Design review of the part built by this model. Coordinates are the model's own, in mm. A direction names the side the tool comes from. Give positions to 0.01 mm unless a question says otherwise; leave off trailing zeros. Loops run counter-clockwise (first coordinate to the right, second up) from the corner with the lowest first, then second, coordinate; pieces in that order, holes last. Notation, with made-up numbers: M 39.5,21.5 L 89.5,21.5 A20 cw 89.5,25.5 Z; hole C -28,-30.75 d1. An arc over 180 degrees is marked long. Answer as CSV lines item,"result".
```python
from build123d import *

# Parameters (mm, degrees)
BOSS_EXTRUDE1_DEPTH = 75
BOSS_EXTRUDE2_START = 225
BOSS_EXTRUDE2_DEPTH = 75
BOSS_EXTRUDE4_START = 75
BOSS_EXTRUDE4_DEPTH = 75
BOSS_EXTRUDE5_DEPTH = 75


# Read off the part's stored shape, not the designer's step: Boss-Extrude4
with BuildPart() as part:
    # Sketch2 → Boss-Extrude1 (new body)
    with BuildSketch(Plane(origin=(0, 0, 0), x_dir=(1, 0, 0), z_dir=(0, 1, 0))):
        with BuildLine():
            ThreePointArc((45, 244.20687951), (47.800691376, 236.146227949), (54.996015936, 231.558714436))
            ThreePointArc((54.996015936, 231.558714436), (116.038816401, 207.795555988), (168.291413922, 168.291413922))
            Line((168.291413922, 168.291413922), (141.421356237, 141.421356237))
            ThreePointArc((141.421356237, 141.421356237), (0, 200), (-141.421356237, 141.421356237))
            Line((-141.421356237, 141.421356237), (-168.291413922, 168.291413922))
            ThreePointArc((-168.291413922, 168.291413922), (-116.038816401, 207.795555988), (-54.996015936, 231.558714436))
            ThreePointArc((-54.996015936, 231.558714436), (-47.800691376, 236.146227949), (-45, 244.20687951))
            Line((-45, 244.20687951), (-45, 275))
            Line((-45, 275), (45, 275))
            Line((45, 275), (45, 244.20687951))
        make_face()
    extrude(amount=BOSS_EXTRUDE1_DEPTH)



with BuildPart() as body_2:
    # Sketch2_3 → Boss-Extrude2 (new body)
    with BuildSketch(Plane(origin=(0, 0, 0), x_dir=(1, 0, 0), z_dir=(0, 1, 0)).offset(BOSS_EXTRUDE2_START)):
        with BuildLine():
            Line((141.421356237, 141.421356237), (168.291413922, 168.291413922))
            ThreePointArc((168.291413922, 168.291413922), (116.038816401, 207.795555988), (54.996015936, 231.558714436))
            ThreePointArc((54.996015936, 231.558714436), (47.800691376, 236.146227949), (45, 244.20687951))
            Line((45, 244.20687951), (45, 275))
            Line((45, 275), (-45, 275))
            Line((-45, 275), (-45, 244.20687951))
            ThreePointArc((-45, 244.20687951), (-47.800691376, 236.146227949), (-54.996015936, 231.558714436))
            ThreePointArc((-54.996015936, 231.558714436), (-116.038816401, 207.795555988), (-168.291413922, 168.291413922))
            Line((-168.291413922, 168.291413922), (-141.421356237, 141.421356237))
            ThreePointArc((-141.421356237, 141.421356237), (0, 200), (141.421356237, 141.421356237))
        make_face()
    extrude(amount=-BOSS_EXTRUDE2_DEPTH)


with BuildPart() as part_1:
    add(part.part)

    add(body_2.part)  # Boss-Extrude4 merges body 2
    # Boss-Extrude4 outline → Boss-Extrude4 (add)
    with BuildSketch(Plane(origin=(0, 0, 0), x_dir=(1, 0, 0), z_dir=(0, 1, 0)).offset(BOSS_EXTRUDE4_START)):
        with BuildLine():
            Line((45, 194.871752699), (45, 275))
            Line((45, 275), (-45, 275))
            Line((-45, 275), (-45, 194.871752699))
            ThreePointArc((-45, 194.871752699), (0, 200), (45, 194.871752699))
        make_face()
    extrude(amount=BOSS_EXTRUDE4_DEPTH)

    # Sketch4_6 → Boss-Extrude5 (add)
    with BuildSketch(Plane(origin=(0, 0, -275), x_dir=(-1, 0, 0), z_dir=(0, 0, -1))):
        with BuildLine():
            ThreePointArc((37.5, 169), (-9.845373608, 205.18450799), (-32.330326321, 150))
            Line((-32.330326321, 150), (32.330326321, 150))
            ThreePointArc((32.330326321, 150), (36.18450799, 159.154626392), (37.5, 169))
        make_face()
        with BuildLine():
            Line((32.330326321, 150), (-32.330326321, 150))
            ThreePointArc((-32.330326321, 150), (0, 131.5), (32.330326321, 150))
        make_face()
        with BuildLine():
            ThreePointArc((32.330326321, 75), (0, 93.5), (-32.330326321, 75))
            Line((-32.330326321, 75), (32.330326321, 75))
        make_face()
        with BuildLine():
            Line((32.330326321, 75), (-32.330326321, 75))
            ThreePointArc((-32.330326321, 75), (-9.845373608, 19.81549201), (37.5, 56))
            ThreePointArc((37.5, 56), (36.18450799, 65.845373608), (32.330326321, 75))
        make_face()
    extrude(amount=BOSS_EXTRUDE5_DEPTH)


solid = part_1.part
```
1. We need section A-A, the plane x = 62. Write out the cut boundary in (y, z), plus the area to 3 significant figures.
Answer block:
outline,"M 0,-229.78 L 75,-229.78 L 75,-190.15 L 0,-190.15 Z; M 150,-229.78 L 225,-229.78 L 225,-190.15 L 150,-190.15 Z"
area,"5,950 mm²"
2. To check wall thickness, follow L1, parallel to Y at x = -10.5, z = -304; L2, parallel to X at y = 28, z = -169.5; L3, parallel to X at y = 97.5, z = -264.5. State the ranges of each line that lie inside material, in increasing order. Write a range as [from, to].
Answer block:
L1,"[20, 92], [133, 205]"
L2,"[-167.07, -106.16], [106.16, 167.07]"
L3,"[-45, 45]"
3. The part is to be moulded in two halves that separate along Y. For faces 1 (the flat face through (-2, 225, -209)), 2 (the flat face through (108, 75, -194)), 3 (the flat face through (2, 0, -209)), 4 (the flat face through (-155, 37, -155)), say which applies: pulls with the +Y half, pulls with the -Y half, needs draft (parallel to the pull), parting line crosses it, or undercut.
Answer block:
face 1,"pulls with the +Y half"
face 2,"undercut"
face 3,"pulls with the -Y half"
face 4,"needs draft"
4. We need section C-C, the plane y = 70. Write out the cut boundary in (x, z).
Answer block:
outline,"M -168.29,-168.29 A238 ccw -55,-231.56 A13 cw -45,-244.21 L -45,-275 L -34.79,-275 L -34.79,-350 L 34.79,-350 L 34.79,-275 L 45,-275 L 45,-244.21 A13 cw 55,-231.56 A238 ccw 168.29,-168.29 L 141.42,-141.42 A200 cw -141.42,-141.42 Z"
5. We need section D-D, the plane x = 0. Write out the cut boundary in (y, z), plus the area to 3 significant figures.
Answer block:
outline,"M 0,-275 L 18.5,-275 L 18.5,-350 L 93.5,-350 L 93.5,-275 L 131.5,-275 L 131.5,-350 L 206.5,-350 L 206.5,-275 L 225,-275 L 225,-200 L 0,-200 Z"
area,"28,100 mm²"
6. We need section B-B, the plane z = -283. Write out the cut boundary in (x, y), plus the area to 3 significant figures.
Answer block:
outline,"C 0,56 d75; C 0,169 d75"
area,"8,840 mm²"
7. For P1, Ø2, axis at y = 160.5, z = -201.5, coming from the -X side; P2, Ø4, axis at y = 59, z = -326.5, coming from the +X side; P3, Ø3, axis at y = 45.5, z = -244.5, coming from the +X side; P4, Ø5, axis at x = 116.5, z = -198, coming from the -Y side, all flat-tipped, find the tip position at first contact; note any pin that passes through.
Answer block:
P1,"x = -128.23"
P2,"x = 37.49"
P3,"x = 45.06"
P4,"y = 0"
8. For faces 5 (the flat face through (-108, 150, -194)), 6 (the flat face through (106, 150, -194)), 7 (the flat face through (45, 111, -243)), 8 (the flat face through (1, 114, -275)), list the 3-axis set-ups (+Z, -Z, +X, -X, +Y, -Y) from which the entire face can be reached by the end or side of a thin tool; tool diameter is ignored.
Answer block:
face 5,"+Z, -Z, -X"
face 6,"+Z, -Z, +X"
face 7,"-Z, +X"
face 8,"-Z"
